Source: CAD feature listing. Evaluate the final solid. Frame: model axes, mm. Face numbers are marked on the shaded views. A direction names the side the tool comes from. Round coordinates to 2 decimals unless told otherwise and drop trailing zeros. Write each loop counter-clockwise with the first axis right and the second up, starting at its lowest first coordinate (ties: lowest second). Pieces come first, ordered by that corner, then holes. Notation, with made-up numbers: M 35,33 L 63,33 A17 cw 63,54 Z; hole C 14.25,-8 d10. An arc over 180 degrees is marked long. Use a Markdown table: item, result.
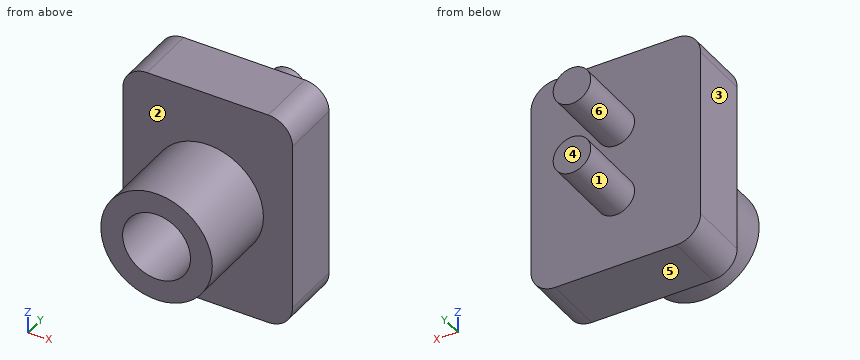
```python
from build123d import *

# Parameters (mm, degrees)
SKETCH1_R           = 4.6
SKETCH1_R_2         = 2.8
ACOPLE_PALITO_DEPTH = 7
CUERPO_START        = 7
SKETCH1_3_W         = 14
SKETCH1_3_H         = 18
SKETCH1_3_R         = 4.6
SKETCH1_3_R_2       = 2.8
CUERPO_DEPTH        = 5
SKETCH2_R           = 1.55
ACOPLE_SENSOR_DEPTH = 6
FILLET1_R           = 2


with BuildPart() as part:
    # Sketch1 → Acople palito (new body)
    with BuildSketch(Plane(origin=(0, 0, 0), x_dir=(1, 0, 0), z_dir=(0, 1, 0))):
        Circle(SKETCH1_R)
        Circle(SKETCH1_R_2, mode=Mode.SUBTRACT)
    extrude(amount=ACOPLE_PALITO_DEPTH)

    # Sketch1_3 → Cuerpo (add)
    with BuildSketch(Plane(origin=(0, 0, 0), x_dir=(1, 0, 0), z_dir=(0, 1, 0)).offset(CUERPO_START)):
        Rectangle(SKETCH1_3_W, SKETCH1_3_H)
        Circle(SKETCH1_3_R, mode=Mode.SUBTRACT)
        Circle(SKETCH1_3_R)
        Circle(SKETCH1_3_R_2, mode=Mode.SUBTRACT)
        Circle(SKETCH1_3_R_2)
    extrude(amount=CUERPO_DEPTH)

    # Sketch2 → Acople sensor (add)
    with BuildSketch(Plane(origin=(0, 12, 0), x_dir=(1, 0, 0), z_dir=(0, 1, 0))):
        with Locations((0, 3)):
            Circle(SKETCH2_R)
        with Locations((0, -3)):
            Circle(SKETCH2_R)
    extrude(amount=ACOPLE_SENSOR_DEPTH)

    # Fillet1
    fillet1_edges = [part.edges().sort_by_distance(p)[0] for p in [
        (-7, 9.5, -9),
        (-7, 9.5, 9),
        (7, 9.5, 9),
        (7, 9.5, -9),
    ]]
    fillet(fillet1_edges, radius=FILLET1_R)


solid = part.part
```
Q1. Line query: L1, parallel to X at y = 2.5, z = 0; L2, parallel to Y at x = -2, z = 2.75. Output: solid intervals per line, ascending.
Results are:
| item | result |
|---|---|
| L1 | -4.6 to -2.8, 2.8 to 4.6 |
| L2 | 0 to 12 |
Q2. Section A-A on x = 0. Return loops of the section in (y, z), plus the area to 3 significant figures.
Results are:
| item | result |
|---|---|
| outline | M 0,-4.6 L 7,-4.6 L 7,-9 L 12,-9 L 12,-4.55 L 18,-4.55 L 18,-1.45 L 12,-1.45 L 12,1.45 L 18,1.45 L 18,4.55 L 12,4.55 L 12,9 L 7,9 L 7,4.6 L 0,4.6 L 0,2.8 L 7,2.8 L 7,-2.8 L 0,-2.8 Z |
| area | 152 mm^2 |
Q3. Section B-B on z = 0. Return loops of the section in (x, y).
Results are:
| item | result |
|---|---|
| outline | M -7,7 L -4.6,7 L -4.6,0 L -2.8,0 L -2.8,7 L 2.8,7 L 2.8,0 L 4.6,0 L 4.6,7 L 7,7 L 7,12 L -7,12 Z |
Q4. First-contact query: pin 1 Ø1 at (x, z) = (1, 6) entering from +Y; pin 2 Ø1.5 at (y, z) = (6, -7) entering from +X; pin 3 Ø1 at (x, y) = (-2.5, 3) entering from -Z; pin 4 Ø1.5 at (x, z) = (-5, 4.5) entering from -Y. Flat tips, straight axial feed; report the tip coordinate or a pass-through.
Results are:
| item | result |
|---|---|
| pin 1 | y = 12 |
| pin 2 | through |
| pin 3 | z = -4.14 |
| pin 4 | y = 7 |
Q5. Reachability of the marked faces 1, 2 and 3 from +Z, -Z, +X, -X, +Y, -Y: full face, straight path, thin tool, end or side. Return the list, or none.
Results are:
| item | result |
|---|---|
| face 1 | +Y |
| face 2 | -Y |
| face 3 | +Z, -Z, -X, +Y, -Y |
Q6. Section D-D on y = 3. Return loops of the section in (x, z), plus the area to 3 significant figures.
Results are:
| item | result |
|---|---|
| outline | C 0,0 d9.2; hole C 0,0 d5.6 |
| area | 41.8 mm^2 |
Q7. Section C-C on y = 16. Return loops of the section in (x, z), plus the area to 3 significant figures.
Results are:
| item | result |
|---|---|
| outline | C 0,-3 d3.1; C 0,3 d3.1 |
| area | 15.1 mm^2 |
Q8. Mould query, pull axis Z, two halves, no side actions, for the marked faces 4, 5 and 6. Classes: +Z half, -Z half, draft (parallel to the pull), parting line (faces both ways), or undercut.
Results are:
| item | result |
|---|---|
| face 4 | draft |
| face 5 | -Z half |
| face 6 | undercut |
